```python
from build123d import *

# Parameters (mm, degrees)
BOSS_EXTRUDE1_DEPTH  = 3.5
SKETCH2_R            = 1.8
SKETCH2_R_2          = 3.920136022
CUT_EXTRUDE1_DEPTH   = 4
SKETCH3_R            = 15
BOSS_EXTRUDE2_DEPTH  = 3.5
SKETCH4_R            = 15
BOSS_EXTRUDE3_DEPTH  = 65
CUT_EXTRUDE2_DEPTH   = 45
BOSS_EXTRUDE4_DEPTH  = 3.5
SKETCH8_R            = 18.202220901
BOSS_EXTRUDE5_DEPTH  = 16
SKETCH9_R            = 15.776157057
SKETCH9_R_2          = 14
CUT_EXTRUDE3_DEPTH   = 49
BOSS_EXTRUDE6_DEPTH  = 3.5
BOSS_EXTRUDE7_DEPTH  = 3.5
SKETCH13_W           = 46.127934492
SKETCH13_H           = 9.661927398
BOSS_EXTRUDE8_DEPTH  = 3.5
SKETCH14_W           = 44.39062698
SKETCH14_H           = 15.435
BOSS_EXTRUDE9_DEPTH  = 9.2
CUT_EXTRUDE4_REACH   = 14.7
SKETCH15_R           = 1.625
FILLET3_R            = 3
SKETCH16_R           = 15.65
SKETCH16_R_2         = 14
BOSS_EXTRUDE10_DEPTH = 49


with BuildPart() as part:
    # Sketch1 → Boss-Extrude1 (new body)
    with BuildSketch(Plane(origin=(0, 0, 0), x_dir=(1, 0, 0), z_dir=(0, 1, 0))):
        with BuildLine():
            Line((-55.85, 37.5), (55.85, 37.5))
            Line((55.85, 37.5), (55.85, -36))
            ThreePointArc((55.85, -36), (55.410660172, -37.060660172), (54.35, -37.5))
            Line((54.35, -37.5), (-54.35, -37.5))
            ThreePointArc((-54.35, -37.5), (-55.410660172, -37.060660172), (-55.85, -36))
            Line((-55.85, -36), (-55.85, 37.5))
        make_face()
    extrude(amount=BOSS_EXTRUDE1_DEPTH)

    # Sketch2 → Cut-Extrude1 (cut)
    with BuildSketch(Plane(origin=(0, 3.5, 0), x_dir=(1, 0, 0), z_dir=(0, 1, 0))):
        with Locations((-42.65, -26.10257403)):
            Circle(SKETCH2_R)
        with Locations((-26.65, -26.10257403)):
            Circle(SKETCH2_R)
        with Locations((26.65, -26.10257403)):
            Circle(SKETCH2_R)
        with Locations((42.65, -26.10257403)):
            Circle(SKETCH2_R)
        with Locations((-50.62881184, 17.336768313)):
            Circle(SKETCH2_R_2)
        with Locations((50.62881184, 17.336768313)):
            Circle(SKETCH2_R_2)
        with BuildLine():
            Line((-16.275049205, -37.5), (-16.275049205, -21.409694211))
            ThreePointArc((-16.275049205, -21.409694211), (0, -5.134645006), (16.275049205, -21.409694211))
            Line((16.275049205, -21.409694211), (16.275049205, -37.5))
            Line((16.275049205, -37.5), (-16.275049205, -37.5))
        make_face()
    extrude(amount=-CUT_EXTRUDE1_DEPTH, mode=Mode.SUBTRACT)

    # Sketch3 → Boss-Extrude2 (add)
    with BuildSketch(Plane(origin=(0, 0, 0), x_dir=(1, 0, 0), z_dir=(0, 1, 0))):
        with Locations((53.706623558, 48.104964972)):
            Circle(SKETCH3_R)
    extrude(amount=BOSS_EXTRUDE2_DEPTH)

    # Sketch4 → Boss-Extrude3 (add)
    with BuildSketch(Plane(origin=(0, 3.5, 0), x_dir=(1, 0, 0), z_dir=(0, 1, 0))):
        with Locations((53.706623558, 48.104964972)):
            Circle(SKETCH4_R)
    extrude(amount=BOSS_EXTRUDE3_DEPTH)

    # Sketch5 → Cut-Extrude2 (cut)
    with BuildSketch(Plane(origin=(0, 68.5, 0), x_dir=(1, 0, 0), z_dir=(0, 1, 0))):
        with BuildLine():
            Line((42.161722237, 46.604964972), (52.206623558, 46.604964972))
            Line((52.206623558, 46.604964972), (52.206623558, 36.560063651))
            ThreePointArc((52.206623558, 36.560063651), (45.474529459, 39.872870873), (42.161722237, 46.604964972))
        make_face()
        with BuildLine():
            Line((65.251524879, 46.604964972), (55.206623558, 46.604964972))
            Line((55.206623558, 46.604964972), (55.206623558, 36.560063651))
            ThreePointArc((55.206623558, 36.560063651), (61.938717657, 39.872870873), (65.251524879, 46.604964972))
        make_face()
        with BuildLine():
            Line((55.206623558, 49.604964972), (65.251524879, 49.604964972))
            ThreePointArc((65.251524879, 49.604964972), (61.938717657, 56.337059071), (55.206623558, 59.649866293))
            Line((55.206623558, 59.649866293), (55.206623558, 49.604964972))
        make_face()
        with BuildLine():
            Line((52.206623558, 59.649866293), (52.206623558, 49.604964972))
            Line((52.206623558, 49.604964972), (42.161722237, 49.604964972))
            ThreePointArc((42.161722237, 49.604964972), (45.474529459, 56.337059071), (52.206623558, 59.649866293))
        make_face()
    extrude(amount=-CUT_EXTRUDE2_DEPTH, mode=Mode.SUBTRACT)

    # Sketch7 → Boss-Extrude4 (add)
    with BuildSketch(Plane(origin=(0, 0, 0), x_dir=(1, 0, 0), z_dir=(0, 1, 0))):
        with BuildLine():
            Line((-12.477353441, 37.5), (55.85, 37.5))
            Line((55.85, 37.5), (55.85, -22.727213829))
            ThreePointArc((55.85, -22.727213829), (59.401653411, 7.516004094), (68.962444737, 36.427208523))
            ThreePointArc((68.962444737, 36.427208523), (65.011720609, 63.638955321), (37.903565045, 59.030779228))
            ThreePointArc((37.903565045, 59.030779228), (14.699548646, 43.617215299), (-12.477353441, 37.5))
        make_face()
    extrude(amount=BOSS_EXTRUDE4_DEPTH)

    # Sketch8 → Boss-Extrude5 (add)
    with BuildSketch(Plane(origin=(0, 3.5, 0), x_dir=(1, 0, 0), z_dir=(0, 1, 0))):
        with Locations((53.706623558, 48.104964972)):
            Circle(SKETCH8_R)
    extrude(amount=BOSS_EXTRUDE5_DEPTH)

    # Sketch9 → Cut-Extrude3 (cut)
    with BuildSketch(Plane(origin=(0, 68.5, 0), x_dir=(1, 0, 0), z_dir=(0, 1, 0))):
        with Locations((53.706623558, 48.104964972)):
            Circle(SKETCH9_R)
        with Locations((53.706623558, 48.104964972)):
            Circle(SKETCH9_R_2, mode=Mode.SUBTRACT)
    extrude(amount=-CUT_EXTRUDE3_DEPTH, mode=Mode.SUBTRACT)

    # Sketch11 → Boss-Extrude6 (add)
    with BuildSketch(Plane(origin=(0, 0, 0), x_dir=(1, 0, 0), z_dir=(0, 1, 0))):
        Polygon((-55.85, 37.5), (-67.841357128, 37.5), (-72.841357128, 37.5), (-72.841357128, 32.5), (-72.841357128, -9.63182819), (-72.841357128, -15.63182819), (-66.841357128, -15.63182819), (-55.85, -15.63182819), (-55.85, -14.63182819), (-55.85, 0), align=None)
    extrude(amount=BOSS_EXTRUDE6_DEPTH)

    # Sketch12 → Boss-Extrude7 (add)
    with BuildSketch(Plane(origin=(0, 3.5, 0), x_dir=(1, 0, 0), z_dir=(0, 1, 0))):
        Polygon((-28.491357128, 15.210034265), (-26.741357128, 15.210034265), (-26.741357128, -13.861045819), (-72.241357128, -13.861045819), (-72.241357128, 13.92894421), (-71.491357128, 13.92894421), (-70.491357128, 13.92894421), (-70.491357128, -12.111045819), (-28.491357128, -12.111045819), align=None)
    extrude(amount=BOSS_EXTRUDE7_DEPTH)

    # Sketch13 → Boss-Extrude8 (add)
    with BuildSketch(Plane(origin=(0, 0, 0), x_dir=(1, 0, 0), z_dir=(0, 1, 0))):
        with Locations((-49.777389882, 42.330963699)):
            Rectangle(SKETCH13_W, SKETCH13_H)
    extrude(amount=BOSS_EXTRUDE8_DEPTH)

    # Sketch14 → Boss-Extrude9 (add)
    with BuildSketch(Plane(origin=(0, 3.5, 0), x_dir=(1, 0, 0), z_dir=(0, 1, 0))):
        with Locations((-50.646043638, 39.444427398)):
            Rectangle(SKETCH14_W, SKETCH14_H)
    extrude(amount=BOSS_EXTRUDE9_DEPTH)

    # Sketch15 → Cut-Extrude4 (cut, up to next)
    with BuildSketch(Plane(origin=(0, 12.7, 0), x_dir=(1, 0, 0), z_dir=(0, 1, 0)), mode=Mode.PRIVATE) as cut_extrude4_sk1:
        with Locations((-64.966357128, 41.090370398)):
            Circle(SKETCH15_R)
    cut_extrude4_tool1 = extrude(cut_extrude4_sk1.sketch, amount=-CUT_EXTRUDE4_REACH, mode=Mode.PRIVATE) & part.part
    add(cut_extrude4_tool1.solids().sort_by_distance((-64.966357, 12.7, -41.09037))[0], mode=Mode.SUBTRACT)
    # Sketch15 → Cut-Extrude4 (cut, up to next)
    with BuildSketch(Plane(origin=(0, 12.7, 0), x_dir=(1, 0, 0), z_dir=(0, 1, 0)), mode=Mode.PRIVATE) as cut_extrude4_sk2:
        with Locations((-34.016357128, 41.090370398)):
            Circle(SKETCH15_R)
    cut_extrude4_tool2 = extrude(cut_extrude4_sk2.sketch, amount=-CUT_EXTRUDE4_REACH, mode=Mode.PRIVATE) & part.part
    add(cut_extrude4_tool2.solids().sort_by_distance((-34.016357, 12.7, -41.09037))[0], mode=Mode.SUBTRACT)

    # Fillet3
    fillet3_edges = [part.edges().sort_by_distance(p)[0] for p in [
        (-72.841357128, 6.35, -47.161927398),
    ]]
    fillet(fillet3_edges, radius=FILLET3_R)

    # Sketch16 → Boss-Extrude10 (add)
    with BuildSketch(Plane(origin=(0, 19.5, 0), x_dir=(1, 0, 0), z_dir=(0, 1, 0))):
        with Locations((53.706623558, 48.104964972)):
            Circle(SKETCH16_R)
        with Locations((53.706623558, 48.104964972)):
            Circle(SKETCH16_R_2, mode=Mode.SUBTRACT)
    extrude(amount=BOSS_EXTRUDE10_DEPTH)


solid = part.part
```
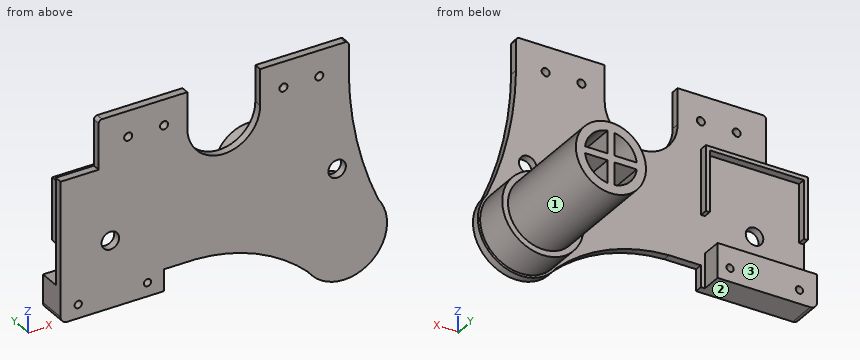
Check sheet for the modelled part. Datum: model origin and axes. Units: mm. Face numbers are marked on the shaded views. A direction names the side the tool comes from. Coordinates: 2 decimals unless noted, no trailing zeros. Write each loop counter-clockwise with the first axis right and the second up, starting at its lowest first coordinate (ties: lowest second). Pieces come first, ordered by that corner, then holes. Notation, with made-up numbers: M 11,65.5 L 49,65.5 A18 cw 49,71.5 Z; hole C 3.5,-14 d3. An arc over 180 degrees is marked long. Write item = value, one per line. Start each with the question number.
1. Thickness scan on probe 1 along X at (y, z) = (41.5, -46.5); probe 2 along Y at (x, z) = (59, -41); probe 3 along Y at (x, z) = (-13, -18.5). Record the ranges inside material, lowest first.
2. Sectioned sample at D-D (z = -9). Record the cut outline in (x, y).
3. Tool access check on the marked faces 1, 2 and 3. Record the directions out of +Z, -Z, +X, -X, +Y, -Y that give a thin tool (end or side, any length) a straight path to the whole face; none if there is none.
4. Go/stop test with flat-tipped pins: pin 1 (10 mm diameter, centred on x = -48.5, y = 14.5, fed in from -Z); pin 2 (4 mm diameter, centred on y = 2.5, z = 32, fed in from +X); pin 3 (12 mm diameter, centred on y = 12, z = -23.5, fed in from +X); pin 4 (12.5 mm diameter, centred on x = -52, z = -42, fed in from +Y). Record where each tip stops, or that it passes through.
5. Sectioned sample at A-A (y = 9.5). Record the cut outline in (x, z) (3 decimals), then the cut area to 3 significant figures.
6. Sectioned sample at C-C (y = 45.5). Record the cut outline in (x, z).
7. Sectioned sample at B-B (x = 26.65). Record the cut outline in (y, z), then the cut area to 3 significant figures.
The answers:
q1.probe_1 = 38.14 to 42.18, 52.21 to 55.21, 65.24 to 69.27
q1.probe_2 = 0 to 23.5
q1.probe_3 = 0 to 3.5
q2.outline = M -72.84,0 L 59.74,0 L 59.74,3.5 L -26.74,3.5 L -26.74,7 L -28.49,7 L -28.49,3.5 L -70.49,3.5 L -70.49,7 L -72.24,7 L -72.24,3.5 L -72.84,3.5 Z
q3.face_1 = +Y
q3.face_2 = -Z, -X, +Y, -Y
q3.face_3 = +Z, -Z, -X, +Y
q4.pin_1 = -47.16
q4.pin_2 = 55.85
q4.pin_3 = through
q4.pin_4 = 12.7
q5.outline = M -72.841,-44.162 A3 ccw -69.841,-47.162 L -28.451,-47.162 L -28.451,-31.727 L -72.841,-31.727 Z; C 53.707,-48.105 d36.404; hole C -64.966,-41.09 d3.25; hole C -34.016,-41.09 d3.25
q5.area = 1,710 mm²
q6.outline = C 53.71,-48.1 d31.3; hole M 42.16,-49.6 A11.64 ccw 52.21,-59.65 L 52.21,-49.6 Z; hole M 42.16,-46.6 L 52.21,-46.6 L 52.21,-36.56 A11.64 ccw Z; hole M 55.21,-59.65 A11.64 ccw 65.25,-49.6 L 55.21,-49.6 Z; hole M 55.21,-46.6 L 65.25,-46.6 A11.64 ccw 55.21,-36.56 Z
q7.outline = M 0,-50.03 L 3.5,-50.03 L 3.5,24.3 L 0,24.3 Z; M 0,27.9 L 3.5,27.9 L 3.5,37.5 L 0,37.5 Z
q7.area = 294 mm²
